Could you check a few things on this model? Use its own coordinates, in mm. A direction names the side the tool comes from. Coordinates: 2 decimals unless noted, no trailing zeros. Order: outer loops, then holes, each group sorted by start corner. A loop starts at its lowest first (then second) coordinate and runs counter-clockwise, first axis right, second up. Notation, with made-up numbers: (6.25, 34) - (49.25, 34) arc R12 ccw to (49.25, 52) - close; hole circle Ø11 at (5, -30.75). An arc over 180 degrees is marked (long way). Answer as a JSON object with one key per item and string values. Group by question number.
(1) Imagine slicing it at C-C, the plane x = -30.48. Write out the boundary of the cut face in (y, z) (3 decimals), and give its area (3 significant figures).
(2) Imagine slicing it at D-D, the plane z = 24.5. Write out the boundary of the cut face in (x, y) (3 decimals), and give its area (3 significant figures).
(3) Imagine slicing it at B-B, the plane y = 7. Write out the boundary of the cut face in (x, z) (3 decimals).
(4) Will these pins go through, and if not, where does the flat tip stop? P1, Ø4, axis at x = -12, y = 8, coming from the -Z side; P2, Ø2.5, axis at x = 18, z = -24.5, coming from the +Y side (3 decimals).
(5) Imagine slicing it at A-A, the plane z = -12. Give the number of separate pieces and of enclosed holes in the cut face, and give its area (3 significant figures).
(6) We'd pull the mould along X, two halves only. Please class faces 4 (the flat face through (-38, 14.445, -25)), 5 (the flat face through (28.575, 2, 0)), 6 (the cylindrical face through (44.14, 2.25, -28.1)), 7 (the cylindrical face through (17.479, 9.375, 28.466)): pulls with the +X half, pulls with the -X half, needs draft (parallel to the pull), parting line crosses it, or undercut.
(7) Which directions (+Z, -Z, +X, -X, +Y, -Y) give clear straight access to the entire face, cutting with the end or side of a thin tool? Please do faces 1 (the flat face through (45, 2, 0)), 2 (the cylindrical face through (10.118, 2.254, 15.875)), 3 (the cylindrical face through (16.987, 9.375, 25.429)).
(8) Please list where these lines run through material, in increasing order: probe 1 along Z at (x, y) = (18, 11) (3 decimals); probe 2 along X at (y, z) = (12, -24.5) (3 decimals); probe 3 along Y at (x, z) = (27, 16.5) (3 decimals).
Autodesk Inventor part; units mm, degrees
ref_plane "YZ Plane" through (0, 0, 0) normal (1, 0, 0) x (0, 1, 0)
ref_plane "XZ Plane" through (0, 0, 0) normal (0, 1, 0) x (-1, 0, 0)
ref_plane "XY Plane" through (0, 0, 0) normal (0, 0, 1) x (1, 0, 0)
sketch "Sketch1" plane through (0, 0, 0) normal (0, 1, 0) x (-1, 0, 0)
  line L0 (-45, -29) -> (45, -29)
  line L1 (45, -29) -> (45, 29)
  line L2 (45, 29) -> (-45, 29)
  line L3 (-45, 29) -> (-45, -29)
  line L4 (-45, -29) -> (45, 29) construction
  line L5 (45, -29) -> (-45, 29) construction
  point P0 (0, 0)
  dimension "d0" = 90
  dimension "d1" = 58
extrude "Extrusion1" add sketch "Sketch1" along normal blind 4.445
fillet "Fillet2" radius 3 4 edges at (45, 2.2225, 29) (-45, 2.2225, 29) (45, 2.2225, -29) (-45, 2.2225, -29)
sketch "Sketch4" plane through (0, 4.445, 0) normal (0, 1, 0) x (1, 0, 0)
  line L0 (0, -13.97) -> (0, 13.97) construction
  line L1 (1.905, -13.97) -> (1.905, 13.97)
  line L2 (-1.905, 13.97) -> (-1.905, -13.97)
  arc A0 (-1.905, -13.97) -> (1.905, -13.97) centre (0, -13.97) ccw
  arc A1 (1.905, 13.97) -> (-1.905, 13.97) centre (0, 13.97) ccw
  line L3 (42, 29) -> (-42, 29) construction
  line L4 (0, 29) -> (0, -29) construction
  line L5 (-42, -29) -> (42, -29) construction
  line L6 (45, -26) -> (45, 26) construction
  line L7 (45, 0) -> (-45, 0) construction
  line L8 (-45, 26) -> (-45, -26) construction
  line L9 (-8.255, -13.97) -> (-8.255, 13.97)
  line L10 (-12.065, 13.97) -> (-12.065, -13.97)
  arc A2 (-8.255, 13.97) -> (-12.065, 13.97) centre (-10.16, 13.97) ccw
  arc A3 (-12.065, -13.97) -> (-8.255, -13.97) centre (-10.16, -13.97) ccw
  line L11 (-18.415, -13.97) -> (-18.415, 13.97)
  line L12 (-22.225, 13.97) -> (-22.225, -13.97)
  arc A4 (-18.415, 13.97) -> (-22.225, 13.97) centre (-20.32, 13.97) ccw
  arc A5 (-22.225, -13.97) -> (-18.415, -13.97) centre (-20.32, -13.97) ccw
  line L13 (-28.575, -13.97) -> (-28.575, 13.97)
  line L14 (-32.385, 13.97) -> (-32.385, -13.97)
  arc A6 (-28.575, 13.97) -> (-32.385, 13.97) centre (-30.48, 13.97) ccw
  arc A7 (-32.385, -13.97) -> (-28.575, -13.97) centre (-30.48, -13.97) ccw
  line L15 (12.065, -13.97) -> (12.065, 13.97)
  line L16 (8.255, 13.97) -> (8.255, -13.97)
  arc A8 (12.065, 13.97) -> (8.255, 13.97) centre (10.16, 13.97) ccw
  arc A9 (8.255, -13.97) -> (12.065, -13.97) centre (10.16, -13.97) ccw
  line L17 (1.905, -13.97) -> (1.905, 13.97)
  line L18 (-1.905, 13.97) -> (-1.905, -13.97)
  arc A10 (1.905, 13.97) -> (-1.905, 13.97) centre (0, 13.97) ccw
  arc A11 (-1.905, -13.97) -> (1.905, -13.97) centre (0, -13.97) ccw
  line L19 (-8.255, -13.97) -> (-8.255, 13.97)
  line L20 (-12.065, 13.97) -> (-12.065, -13.97)
  arc A12 (-8.255, 13.97) -> (-12.065, 13.97) centre (-10.16, 13.97) ccw
  arc A13 (-12.065, -13.97) -> (-8.255, -13.97) centre (-10.16, -13.97) ccw
  line L21 (-18.415, -13.97) -> (-18.415, 13.97)
  line L22 (-22.225, 13.97) -> (-22.225, -13.97)
  arc A14 (-18.415, 13.97) -> (-22.225, 13.97) centre (-20.32, 13.97) ccw
  arc A15 (-22.225, -13.97) -> (-18.415, -13.97) centre (-20.32, -13.97) ccw
  line L23 (22.225, -13.97) -> (22.225, 13.97)
  line L24 (18.415, 13.97) -> (18.415, -13.97)
  arc A16 (22.225, 13.97) -> (18.415, 13.97) centre (20.32, 13.97) ccw
  arc A17 (18.415, -13.97) -> (22.225, -13.97) centre (20.32, -13.97) ccw
  line L25 (12.065, -13.97) -> (12.065, 13.97)
  line L26 (8.255, 13.97) -> (8.255, -13.97)
  arc A18 (12.065, 13.97) -> (8.255, 13.97) centre (10.16, 13.97) ccw
  arc A19 (8.255, -13.97) -> (12.065, -13.97) centre (10.16, -13.97) ccw
  line L27 (1.905, -13.97) -> (1.905, 13.97)
  line L28 (-1.905, 13.97) -> (-1.905, -13.97)
  arc A20 (1.905, 13.97) -> (-1.905, 13.97) centre (0, 13.97) ccw
  arc A21 (-1.905, -13.97) -> (1.905, -13.97) centre (0, -13.97) ccw
  line L29 (-8.255, -13.97) -> (-8.255, 13.97)
  line L30 (-12.065, 13.97) -> (-12.065, -13.97)
  arc A22 (-8.255, 13.97) -> (-12.065, 13.97) centre (-10.16, 13.97) ccw
  arc A23 (-12.065, -13.97) -> (-8.255, -13.97) centre (-10.16, -13.97) ccw
  line L31 (32.385, -13.97) -> (32.385, 13.97)
  line L32 (28.575, 13.97) -> (28.575, -13.97)
  arc A24 (32.385, 13.97) -> (28.575, 13.97) centre (30.48, 13.97) ccw
  arc A25 (28.575, -13.97) -> (32.385, -13.97) centre (30.48, -13.97) ccw
  line L33 (22.225, -13.97) -> (22.225, 13.97)
  line L34 (18.415, 13.97) -> (18.415, -13.97)
  arc A26 (22.225, 13.97) -> (18.415, 13.97) centre (20.32, 13.97) ccw
  arc A27 (18.415, -13.97) -> (22.225, -13.97) centre (20.32, -13.97) ccw
  line L35 (12.065, -13.97) -> (12.065, 13.97)
  line L36 (8.255, 13.97) -> (8.255, -13.97)
  arc A28 (12.065, 13.97) -> (8.255, 13.97) centre (10.16, 13.97) ccw
  arc A29 (8.255, -13.97) -> (12.065, -13.97) centre (10.16, -13.97) ccw
  line L37 (1.905, -13.97) -> (1.905, 13.97)
  line L38 (-1.905, 13.97) -> (-1.905, -13.97)
  arc A30 (1.905, 13.97) -> (-1.905, 13.97) centre (0, 13.97) ccw
  arc A31 (-1.905, -13.97) -> (1.905, -13.97) centre (0, -13.97) ccw
  point P0 (0, 0)
  dimension "d18" = 13.97
  dimension "d19" = 3.81
  dimension "d22" = 10.16
  dimension "d25" = 10.16
extrude "Extrusion3" cut sketch "Sketch4" against normal blind 4.445
sketch "Sketch5" plane through (0, 4.445, 0) normal (0, 1, 0) x (1, 0, 0)
  circle A0 centre (-40, 24.5) radius 4
  circle A1 centre (-40, 24.5) radius 1.375
  line L0 (-45, 26) -> (-45, -26)
  line L1 (42, 29) -> (-42, 29)
  line L2 (-45, 0) -> (45, 0)
  line L3 (45, -26) -> (45, 26)
  circle A2 centre (-40, -24.5) radius 4
  circle A3 centre (-40, -24.5) radius 1.375
  circle A4 centre (18, 24.5) radius 4
  circle A5 centre (18, 24.5) radius 1.375
  circle A6 centre (18, -24.5) radius 4
  circle A7 centre (18, -24.5) radius 1.375
  line L4 (-42, -29) -> (42, -29)
  point P0 (0, 0)
  dimension "d35" = 8
  dimension "d36" = 2.75
  dimension "d37" = 5
  dimension "d39" = 8
  dimension "d40" = 2.75
  dimension "d41" = 58
  dimension "d43" = 4.5
  dimension "d45" = 8
  dimension "d46" = 2.75
  dimension "d47" = 49
  dimension "d50" = 58
  dimension "d51" = 4.5
extrude "Extrusion4" add sketch "Sketch5" along normal blind 10
properties part number "_3DPrint"
Result set:
{
 "1": {"outline": "(0, -29) - (4.445, -29) - (4.445, -15.875) - (0, -15.875) - close; (0, 15.875) - (4.445, 15.875) - (4.445, 29) - (0, 29) - close", "area": "117 mm^2"},
 "2": {"outline": "(-45, 0) - (45, 0) - (45, 4.445) - (22, 4.445) - (22, 14.445) - (19.375, 14.445) - (19.375, 4.445) - (16.625, 4.445) - (16.625, 14.445) - (14, 14.445) - (14, 4.445) - (-36, 4.445) - (-36, 14.445) - (-38.625, 14.445) - (-38.625, 4.445) - (-41.375, 4.445) - (-41.375, 14.445) - (-44, 14.445) - (-44, 4.445) - (-45, 4.445) - close", "area": "505 mm^2"},
 "3": {"outline": "circle Ø8 at (-40, -24.5); circle Ø8 at (-40, 24.5); circle Ø8 at (18, -24.5); circle Ø8 at (18, 24.5); hole circle Ø2.75 at (-40, -24.5); hole circle Ø2.75 at (-40, 24.5); hole circle Ø2.75 at (18, -24.5); hole circle Ø2.75 at (18, 24.5)"},
 "4": {"P1": "passes through", "P2": "stops at y = 4.445"},
 "5": {"separate pieces": "8", "enclosed holes": "0", "area": "282 mm^2"},
 "6": {"face 4": "needs draft", "face 5": "undercut", "face 6": "pulls with the +X half", "face 7": "undercut"},
 "7": {"face 1": "+Z, -Z, +X, +Y, -Y", "face 2": "+Y, -Y", "face 3": "+Y"},
 "8": {"probe 1": "z = -28.5 to -25.875, -23.125 to -20.5, 20.5 to 23.125, 25.875 to 28.5", "probe 2": "x = -44 to -41.375, -38.625 to -36, 14 to 16.625, 19.375 to 22", "probe 3": "y = 0 to 4.445"}
}
